Could you check a few things on this model? Use its own coordinates, in mm. A direction names the side the tool comes from. Round coordinates to 2 decimals unless told otherwise and drop trailing zeros. Loops run counter-clockwise (first coordinate to the right, second up) from the corner with the lowest first, then second, coordinate; pieces in that order, holes last. Notation, with made-up numbers: (-25.5, 12) - (24.5, 12) arc R24 cw to (24.5, 51) - close; hole circle Ø9 at (43, 63). An arc over 180 degrees is marked (long way). Use one line per item in the form item = value.
```python
from build123d import *

# Parameters (mm, degrees)
BOSS_EXTRUDE3_DEPTH = 22
FILLET2_R           = 10
SHELL1_T            = -3
BOSS_EXTRUDE4_DEPTH = 2
SKETCH4_R           = 5
BOSS_EXTRUDE5_DEPTH = 11


with BuildPart() as part:
    # Sketch2 → Boss-Extrude3 (new body)
    with BuildSketch(Plane.XY):
        with BuildLine():
            Line((0, 0), (0, 64))
            Line((0, 64), (19, 64))
            ThreePointArc((19, 64), (51, 32), (19, 0))
            Line((19, 0), (0, 0))
        make_face()
    extrude(amount=BOSS_EXTRUDE3_DEPTH)

    # Fillet2
    fillet2_edges = [part.edges().sort_by_distance(p)[0] for p in [
        (9.5, 64, 22),
        (9.5, 0, 22),
        (51, 32, 22),
    ]]
    fillet(fillet2_edges, radius=FILLET2_R)

    # Shell1
    shell1_openings = [part.faces().sort_by_distance(p)[0] for p in [
        (17.5, 32, 0),
    ]]
    offset(amount=SHELL1_T, openings=shell1_openings, kind=Kind.INTERSECTION)

    # Sketch3 → Boss-Extrude4 (add)
    with BuildSketch(Plane(origin=(0, 0, 0), x_dir=(-1, 0, 0), z_dir=(0, 0, -1))):
        with BuildLine():
            Line((2, -2), (2, 66))
            Line((2, 66), (-19, 66))
            ThreePointArc((-19, 66), (-53, 32), (-19, -2))
            Line((-19, -2), (2, -2))
        make_face()
        with BuildLine():
            Line((-3, 3), (-3, 61))
            Line((-3, 61), (-19, 61))
            ThreePointArc((-19, 61), (-48, 32), (-19, 3))
            Line((-19, 3), (-3, 3))
        make_face(mode=Mode.SUBTRACT)
    extrude(amount=BOSS_EXTRUDE4_DEPTH)

    # Sketch4 → Boss-Extrude5 (add)
    with BuildSketch(Plane(origin=(0, 0, 19), x_dir=(-1, 0, 0), z_dir=(0, 0, -1))):
        with Locations((-19, 32)):
            Circle(SKETCH4_R)
    extrude(amount=BOSS_EXTRUDE5_DEPTH)


solid = part.part
```
1. If we section it at A-A, the plane z = 0.75: Write out the boundary of the cut face in (x, y).
Solution:
outline = (0, 0) - (19, 0) arc R32 ccw to (19, 64) - (0, 64) - close; hole (3, 3) - (19, 3) arc R29 ccw to (19, 61) - (3, 61) - close
2. If we section it at B-B, the plane z = 18: Write out the boundary of the cut face in (x, y).
Solution:
outline = (0, 2) - (19, 2) arc R30 ccw to (19, 62) - (0, 62) - close; circle Ø10 at (19, 32); hole (3, 6.39) - (19, 6.39) arc R25.61 ccw to (19, 57.61) - (3, 57.61) - close
3. We'd pull the mould along X, two halves only. Please class faces 1 (the face through (-2, 32, -1)), 2 (the face through (47.993, 32.638, 5.098)), 3 (the face through (50.992, 32.704, 5.916)): +X half, -X half, draft (parallel to the pull), parting line (faces both ways), or undercut.
Solution:
face_1 = -X half
face_2 = undercut
face_3 = +X half
4. Please list where these lines run through material, in increasing order: line 1 along Y through (x, z) = (19.5, -0.25); line 2 along X through (y, z) = (31.5, 16); line 3 along Y through (x, z) = (5.5, 9).
Solution:
line_1 = -2 to 3, 61 to 66
line_2 = 0 to 3, 14.03 to 23.97, 46.74 to 50.16
line_3 = 0 to 3, 61 to 64
5. For P1, Ø12, axis at x = 35.5, z = 6.5, coming from the -Y side; P2, Ø4, axis at x = 12.5, z = 5, coming from the +Y side; P3, Ø1, axis at x = 34, z = 19.5, coming from the -Y side; P4, Ø13, axis at x = 10, z = 5.5, coming from the +Y side, each with a flat end and sliding along its axis, tell me the tip position at first contact or that it passes through.
Solution:
P1 = 1.77
P2 = 64
P3 = 6.94
P4 = 66
6. If we section it at C-C, the plane x = 10.5: Write out the boundary of the cut face in (y, z), plus the area to 3 significant figures.
Solution:
outline = (-2, -2) - (3, -2) - (3, 12) arc R7 cw to (10, 19) - (54, 19) arc R7 cw to (61, 12) - (61, -2) - (66, -2) - (66, 0) - (64, 0) - (64, 12) arc R10 ccw to (54, 22) - (10, 22) arc R10 ccw to (0, 12) - (0, 0) - (-2, 0) - close
area = 304 mm^2
7. On a 3-axis mill with a long thin cutter (end or side, diameter ignored), from which of +Z, -Z, +X, -X, +Y, -Y can I reach the whole of each face in a straight line? I mean faces 4 (the face through (9, 64, 6)), 5 (the face through (52.99, 32.75, -0.99)), 6 (the face through (19, 32, 8)), 7 (the face through (0, 32, 11)), 8 (the face through (9, -2, -1)). Say none if no direction works.
Solution:
face_4 = +Z, +X, -X, +Y
face_5 = +Z, -Z, +X
face_6 = -Z
face_7 = +Z, -X, +Y, -Y
face_8 = +Z, -Z, +X, -X, -Y
8. If we section it at D-D, the plane y = 32: Write out the boundary of the cut face in (x, z).
Solution:
outline = (-2, -2) - (3, -2) - (3, 19) - (14, 19) - (14, 8) - (24, 8) - (24, 19) - (41, 19) arc R7 cw to (48, 12) - (48, -2) - (53, -2) - (53, 0) - (51, 0) - (51, 12) arc R10 ccw to (41, 22) - (0, 22) - (0, 0) - (-2, 0) - close
